from build123d import *

# Parameters (mm, degrees)
F1_DEPTH = 15
F2_R     = 4
F3_DEPTH = 5


with BuildPart() as f1:
    # F0 (on Front) → F1 (new body, symmetric)
    with BuildSketch(Plane.XZ):
        with BuildLine():
            Line((0, -50), (50, -50))
            Line((50, -50), (50, 50))
            Line((50, 50), (0, 50))
            Line((0, 50), (0, -15))
            Line((0, -15), (-10.5, -15))
            ThreePointArc((-10.5, -15), (-18, -22.5), (-10.5, -30))
            Line((-10.5, -30), (0, -30))
            Line((0, -30), (0, -50))
        make_face()
    extrude(amount=F1_DEPTH, both=True)

    # F2 (on face) → F3 (cut)
    with BuildSketch(Plane.XZ.offset(15)):
        with Locations((25, 25)):
            Circle(F2_R)
    extrude(amount=-F3_DEPTH, mode=Mode.SUBTRACT)


solid = f1.part
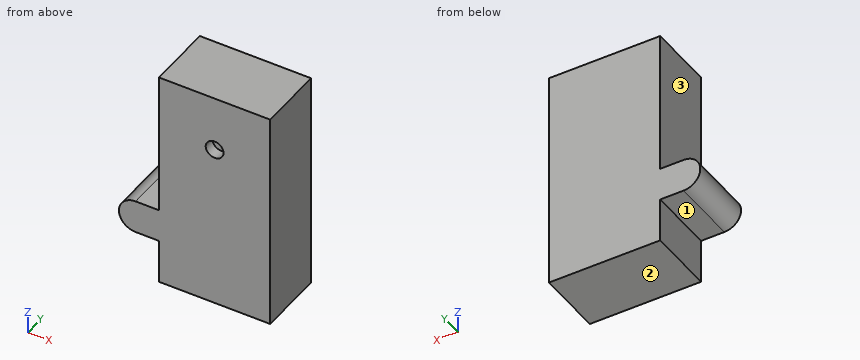
The listing builds one solid part. Answer for the finished solid, in the listing's coordinates (mm). Face numbers are marked on the shaded views. A direction names the side the tool comes from. Round coordinates to 2 decimals unless told otherwise and drop trailing zeros. Write each loop counter-clockwise with the first axis right and the second up, starting at its lowest first coordinate (ties: lowest second). Pieces come first, ordered by that corner, then holes. Notation, with made-up numbers: (76.25, 30) - (116.25, 30) arc R37 ccw to (116.25, 66) - close; hole circle Ø10 at (79.25, 10). An arc over 180 degrees is marked (long way). Use one line per item in the form item = value. Start each with the question number.
Item 1: Find the intervals of material crossed by line 1 (Z direction, x = 25, y = -12.65); line 2 (X direction, y = -10.25, z = -13); line 3 (Z direction, x = -2.5, y = 6.25), in increasing order. Write a range as [from, to].
Item 2: A cutting plane is placed at C-C (y = 1.5). Write down the section's boundary in (x, z), plus the area to 3 significant figures.
Item 3: A cutting plane is placed at D-D (z = -4). Write down the section's boundary in (x, y).
Item 4: A tool of negligible diameter and unlimited length cuts with its end or side. For the marked faces 1, 2 and 3, from which of +Z, -Z, +X, -X, +Y, -Y can it reach the whole face along a straight path? Write none if from no direction.
Item 5: Flat-ended cylindrical pins translate along their axes: pin 1 Ø10 at (y, z) = (5, -40) entering from -X; pin 2 Ø5 at (x, y) = (-7.5, 3.5) entering from -Z; pin 3 Ø5 at (x, y) = (-7, 6) entering from +Z; pin 4 Ø6.5 at (x, z) = (27, 25) entering from -Y. Find the tip coordinate at first contact, or state that the pin passes through.
Item 6: A cutting plane is placed at B-B (z = 25). Write down the section's boundary in (x, y), plus the area to 3 significant figures.
Item 7: A cutting plane is placed at A-A (y = -12.5). Write down the section's boundary in (x, z).
The answers:
q1.line_1 = [-50, 21], [29, 50]
q1.line_2 = [0, 50]
q1.line_3 = [-30, -15]
q2.outline = (-10.5, -30) - (0, -30) - (0, -50) - (50, -50) - (50, 50) - (0, 50) - (0, -15) - (-10.5, -15) arc R7.5 ccw to start
q2.area = 5,250 mm^2
q3.outline = (0, -15) - (50, -15) - (50, 15) - (0, 15) - close
q4.face_1 = -Z, -X, +Y, -Y
q4.face_2 = -Z, +X, -X, +Y, -Y
q4.face_3 = +Z, -X, +Y, -Y
q5.pin_1 = 0
q5.pin_2 = -30
q5.pin_3 = -15
q5.pin_4 = -15
q6.outline = (0, -15) - (21, -15) - (21, -10) - (29, -10) - (29, -15) - (50, -15) - (50, 15) - (0, 15) - close
q6.area = 1,460 mm^2
q7.outline = (-10.5, -30) - (0, -30) - (0, -50) - (50, -50) - (50, 50) - (0, 50) - (0, -15) - (-10.5, -15) arc R7.5 ccw to start; hole circle Ø8 at (25, 25)
